```python
from build123d import *

# Parameters (mm, degrees)
ESQUISSE2_R             = 12
BOSS_EXTRU_1_DEPTH      = 40
ESQUISSE3_W             = 7.8
ESQUISSE3_H             = 4.051853135
BOSS_EXTRU_3_DEPTH      = 40
ESQUISSE4_R             = 9.5
ENL_V_MAT_EXTRU_3_DEPTH = 32
ESQUISSE6_W             = 6
ESQUISSE6_H             = 3.848056491
ENL_V_MAT_EXTRU_4_DEPTH = 32
ESQUISSE7_R             = 3.5
ENL_V_MAT_EXTRU_5_DEPTH = 42


with BuildPart() as part:
    # Esquisse2 → Boss.-Extru.1 (new body)
    with BuildSketch(Plane.XY):
        Circle(ESQUISSE2_R)
    extrude(amount=BOSS_EXTRU_1_DEPTH)

    # Esquisse3 → Boss.-Extru.3 (add)
    with BuildSketch(Plane.XY):
        with Locations((0, 12.974073433)):
            Rectangle(ESQUISSE3_W, ESQUISSE3_H)
    extrude(amount=BOSS_EXTRU_3_DEPTH)

    # Esquisse4 → Enlèv. mat.-Extru.3 (cut)
    with BuildSketch(Plane.XY):
        Circle(ESQUISSE4_R)
    extrude(amount=ENL_V_MAT_EXTRU_3_DEPTH, mode=Mode.SUBTRACT)

    # Esquisse6 → Enlèv. mat.-Extru.4 (cut)
    with BuildSketch(Plane.XY):
        with Locations((0, 10.275971755)):
            Rectangle(ESQUISSE6_W, ESQUISSE6_H)
    extrude(amount=ENL_V_MAT_EXTRU_4_DEPTH, mode=Mode.SUBTRACT)

    # Esquisse7 → Enlèv. mat.-Extru.5 (cut)
    with BuildSketch(Plane.XY):
        Circle(ESQUISSE7_R)
    extrude(amount=ENL_V_MAT_EXTRU_5_DEPTH, mode=Mode.SUBTRACT)


solid = part.part
```
Geometry: final body of the model. Coordinates: model frame, mm. A direction names the side the tool comes from. Round coordinates to 2 decimals unless told otherwise and drop trailing zeros. Write each loop counter-clockwise with the first axis right and the second up, starting at its lowest first coordinate (ties: lowest second). Pieces come first, ordered by that corner, then holes. Notation, with made-up numbers: (6, 22.5) -> (65, 22.5) arc R20 cw to (65, 38.5) -> close; hole circle Ø9 at (-16, -3.75). An arc over 180 degrees is marked (long way). Return JSON: item names as keys, results as strings.
Q1. Section B-B on x = 0. Return the cut outline in (y, z), and give its area (3 significant figures).
From the geometry:
{"outline": "(-12, 0) -> (-9.5, 0) -> (-9.5, 32) -> (-3.5, 32) -> (-3.5, 40) -> (-12, 40) -> close; (3.5, 32) -> (12.2, 32) -> (12.2, 0) -> (15, 0) -> (15, 40) -> (3.5, 40) -> close", "area": "330 mm2"}
Q2. Section A-A on y = 0. Return the cut outline in (x, z).
From the geometry:
{"outline": "(-12, 0) -> (-9.5, 0) -> (-9.5, 32) -> (-3.5, 32) -> (-3.5, 40) -> (-12, 40) -> close; (3.5, 32) -> (9.5, 32) -> (9.5, 0) -> (12, 0) -> (12, 40) -> (3.5, 40) -> close"}
Q3. Ray query, line 1 (X direction, y = 0, z = 38.5); line 2 (X direction, y = 0, z = 21); line 3 (Z direction, x = 7.5, y = -3.75). Return the intervals inside material, ascending.
From the geometry:
{"line 1": "-12 to -3.5, 3.5 to 12", "line 2": "-12 to -9.5, 9.5 to 12", "line 3": "32 to 40"}
Q4. Set-up query: faces 1 (the flat face through (0, 12.2, 16)), 2 (the flat face through (3.9, 13, 20)), 3 (the cylindrical face through (3.233, -1.341, 35.944)). Return all of +Z, -Z, +X, -X, +Y, -Y with unobstructed straight access to the full face (end or side cutting, diameter ignored); none if empty.
From the geometry:
{"face 1": "-Z", "face 2": "+Z, -Z, +X, +Y", "face 3": "+Z, -Z"}
Q5. Mould query, pull axis Y, two halves, no side actions, for faces 4 (the cylindrical face through (0, -12, 20)), 5 (the flat face through (0, 15, 20)), 6 (the cylindrical face through (-0.375, -9.493, 15.776)), 7 (the flat face through (-3.9, 13, 20)). Classes: +Y half, -Y half, draft (parallel to the pull), parting line (faces both ways), or undercut.
From the geometry:
{"face 4": "parting line", "face 5": "+Y half", "face 6": "undercut", "face 7": "draft"}
Q6. First-contact query: pin 1 Ø3 at (y, z) = (13, 21) entering from +X; pin 2 Ø8 at (x, y) = (0, 0) entering from -Z; pin 3 Ø6 at (x, z) = (4.5, 20.5) entering from -Y. Flat tips, straight axial feed; report the tip coordinate or a pass-through.
From the geometry:
{"pin 1": "x = 3.9", "pin 2": "z = 32", "pin 3": "y = -11.91"}
Q7. Section C-C on z = 17. Return the cut outline in (x, y).
From the geometry:
{"outline": "(-3.9, 11.35) arc R12 ccw (long way) to (3.9, 11.35) -> (3.9, 15) -> (-3.9, 15) -> close; hole (-3, 9.01) arc R9.5 ccw (long way) to (3, 9.01) -> (3, 12.2) -> (-3, 12.2) -> close"}
Q8. Section D-D on y = 10.5. Return the cut outline in (x, z), and give its area (3 significant figures).
From the geometry:
{"outline": "(-5.81, 0) -> (-3, 0) -> (-3, 32) -> (3, 32) -> (3, 0) -> (5.81, 0) -> (5.81, 40) -> (-5.81, 40) -> close", "area": "273 mm2"}
